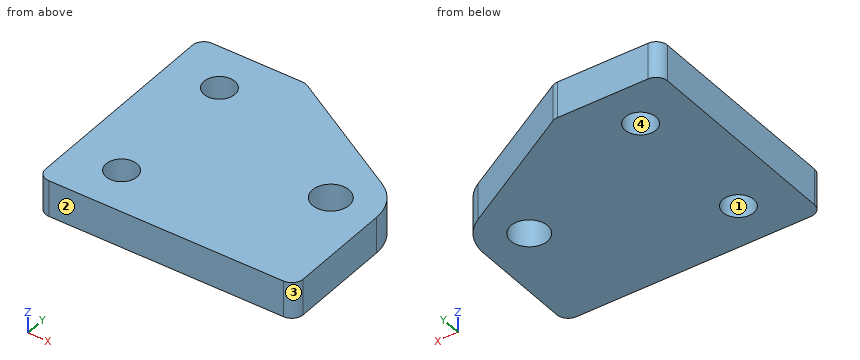
Autodesk Inventor part; units mm, degrees
ref_plane "YZ Plane" through (0, 0, 0) normal (1, 0, 0) x (0, 1, 0)
ref_plane "XZ Plane" through (0, 0, 0) normal (0, 1, 0) x (-1, 0, 0)
ref_plane "XY Plane" through (0, 0, 0) normal (0, 0, 1) x (1, 0, 0)
sketch "Sketch1" plane through (0, 0, 0) normal (0, 0, 1) x (1, 0, 0)
  line L0 (22.5, -20) -> (-22.5, -20)
  line L1 (-22.5, -20) -> (-22.5, 20)
  line L2 (-22.5, 20) -> (22.5, 20)
  line L3 (22.5, 20) -> (22.5, -20)
  line L4 (22.5, -20) -> (-22.5, 20) construction
  line L5 (-22.5, -20) -> (22.5, 20) construction
  circle A0 centre (14.5, 0) radius 8
  line L6 (18.5, 6.9282) -> (-4.141, 20)
  circle A1 centre (-13.5, 12) radius 2.7
  circle A2 centre (-13.5, -12) radius 2.7
  point P0 (0, 0)
  point P1 (22.5, 0)
  dimension "d4" = 16
  dimension "d0" = 40
  dimension "d1" = 9
  dimension "d2" = 8
  dimension "d3" = 8
  dimension "d5" = 28
  dimension "d6" = 30
  dimension "d7" = 20
  dimension "d8" = 5.4
extrude "Extrusion1" add sketch "Sketch1" along normal blind 6.35 contours L0 L1 L2 L6 A0 L3 | A0
sketch "Sketch2" plane through (0, 0, 6.35) normal (0, 0, 1) x (1, 0, 0)
  arc A0 (22.5, 0) -> (18.5, 6.9282) centre (14.5, 0) ccw
  point P0 (0, 0)
hole "Hole1" at (14.5, 0, 6.35) direction (0, 0, -1) diameter 6.4008 end through all
fillet "Fillet1" radius 2 4 edges at (-22.5, 20, 3.175) (-22.5, -20, 3.175) (22.5, -20, 3.175) (-4.141, 20, 3.175)
properties part number "Gas Strut Lower Plate"
Source: CAD feature listing. Evaluate the final solid. Frame: model axes, mm. Face numbers are marked on the shaded views. Coordinates: 2 decimals unless noted, no trailing zeros. Write each loop counter-clockwise with the first axis right and the second up, starting at its lowest first coordinate (ties: lowest second). Pieces come first, ordered by that corner, then holes. Notation, with made-up numbers: (77.25, -37.5) -> (94.25, -37.5) arc R14 cw to (94.25, -18.5) -> close; hole circle Ø5 at (-33, 14). An arc over 180 degrees is marked (long way). Return JSON: item names as keys, results as strings. Group by question number.
1) Section query A-A, the plane x = -13.5. Return loops of the section in (y, z), plus the area to 3 significant figures.
2) Section query C-C, the plane y = -12. Return loops of the section in (x, z).
3) Ray query, line 1 along Y through (x, z) = (-13.5, 2.25); line 2 along Y through (x, z) = (-15, 4.5) (3 decimals); line 3 along X through (y, z) = (11, 1.75). Return the intervals inside material, ascending.
4) Contact query for flat-ended pins moving along their axis: P1, Ø7.5, axis at x = 14.5, y = 0, coming from the +Z side; P2, Ø5, axis at x = -13.5, y = 12, coming from the -Z side; P3, Ø1.5, axis at y = 6.5, z = 1.5, coming from the +X side. Output: stop coordinate, or through.
5) Section query D-D, the plane x = 14.5. Return loops of the section in (y, z).
6) Mould query, pull axis X, two halves, no side actions, for the marked faces 1, 2, 3 and 4. Classes: +X half, -X half, draft (parallel to the pull), parting line (faces both ways), or undercut.
7) Section query B-B, the plane z = 2. Return loops of the section in (x, y), plus the area to 3 significant figures.
From the geometry:
{
 "1": {"outline": "(-20, 0) -> (-14.7, 0) -> (-14.7, 6.35) -> (-20, 6.35) -> close; (-9.3, 0) -> (9.3, 0) -> (9.3, 6.35) -> (-9.3, 6.35) -> close; (14.7, 0) -> (20, 0) -> (20, 6.35) -> (14.7, 6.35) -> close", "area": "185 mm²"},
 "2": {"outline": "(-22.5, 0) -> (-16.2, 0) -> (-16.2, 6.35) -> (-22.5, 6.35) -> close; (-10.8, 0) -> (22.5, 0) -> (22.5, 6.35) -> (-10.8, 6.35) -> close"},
 "3": {"line 1": "-20 to -14.7, -9.3 to 9.3, 14.7 to 20", "line 2": "-20 to -14.245, -9.755 to 9.755, 14.245 to 20", "line 3": "-22.5 to -16.01, -10.99 to 11.45"},
 "4": {"P1": "z = 6.35", "P2": "through", "P3": "x = 20.06"},
 "5": {"outline": "(-20, 0) -> (-3.2, 0) -> (-3.2, 6.35) -> (-20, 6.35) -> close; (3.2, 0) -> (9.24, 0) -> (9.24, 6.35) -> (3.2, 6.35) -> close"},
 "6": {"face 1": "undercut", "face 2": "draft", "face 3": "+X half", "face 4": "undercut"},
 "7": {"outline": "(-22.5, -18) arc R2 ccw to (-20.5, -20) -> (20.5, -20) arc R2 ccw to (22.5, -18) -> (22.5, 0) arc R8 ccw to (18.5, 6.93) -> (-3.68, 19.73) arc R2 ccw to (-4.68, 20) -> (-20.5, 20) arc R2 ccw to (-22.5, 18) -> close; hole circle Ø5.4 at (-13.5, -12); hole circle Ø5.4 at (-13.5, 12); hole circle Ø6.4 at (14.5, 0)", "area": "1,510 mm²"}
}
